Study the drawing (mm; zero at the part's minimum x, y, z) and answer. A direction names the side the tool comes from. Round coordinates to 2 decimals unless told otherwise and drop trailing zeros. Order: outer loops, then holes, each group sorted by start corner. A loop starts at its lowest first (then second) coordinate and runs counter-clockwise, first axis right, second up. Notation, with made-up numbers: (45, -40) -> (64, -40) arc R30 ccw to (64, -5) -> close; hole circle Ø4 at (66, 6). An arc over 180 degrees is marked (long way). Use one line per item in the form item = value.
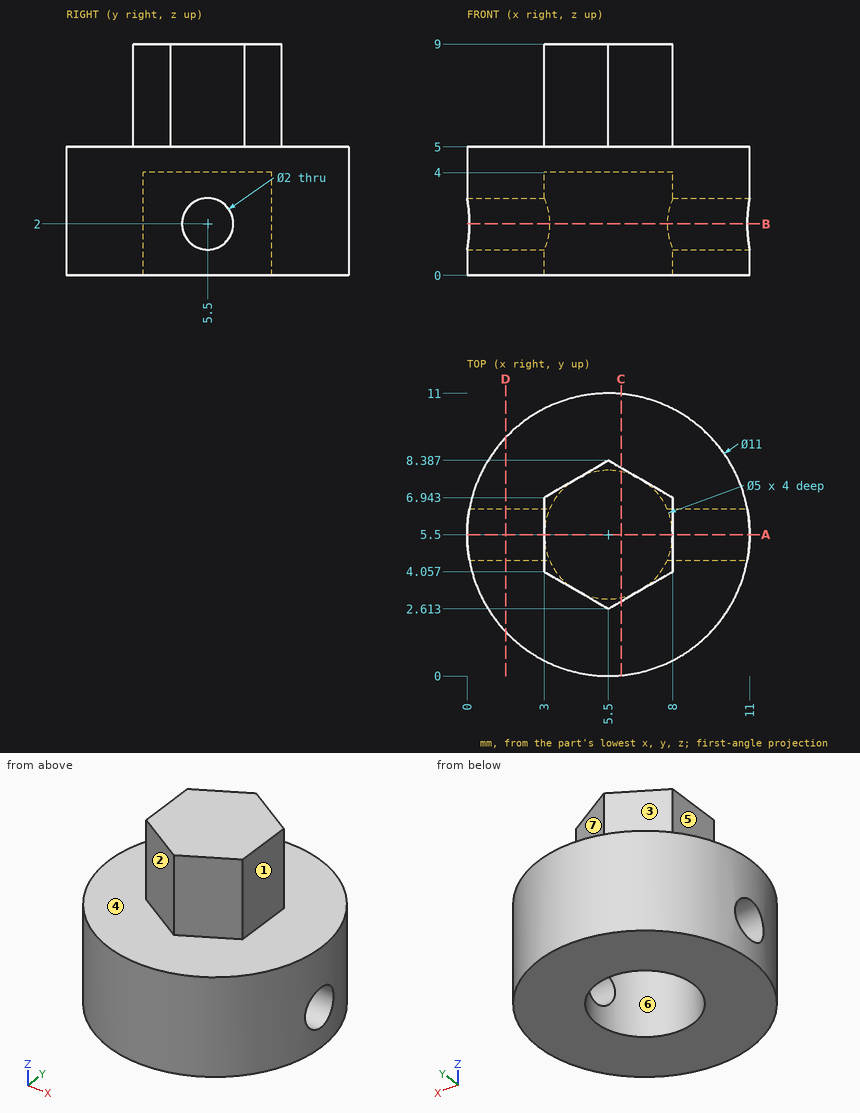
Item 1: Determine the mould class of the marked faces 5, 6 and 7 for opening direction Y: released by +Y, released by -Y, zero draft, split by the parting line, or undercut.
Findings:
face_5 = zero draft
face_6 = undercut
face_7 = released by +Y
Item 2: The part is cut by section A-A, the plane y = 5.5. Give the vertices of the cut face in (x, z), and give its area (3 significant figures).
Findings:
outline = (0, 0) -> (3, 0) -> (3, 1) -> (0, 1) -> close; (0, 3) -> (3, 3) -> (3, 4) -> (8, 4) -> (8, 3) -> (11, 3) -> (11, 5) -> (8, 5) -> (8, 9) -> (3, 9) -> (3, 5) -> (0, 5) -> close; (8, 0) -> (11, 0) -> (11, 1) -> (8, 1) -> close
area = 43.0 mm^2
Item 3: The part is cut by section C-C, the plane x = 6. Give the vertices of the cut face in (y, z).
Findings:
outline = (0.02, 0) -> (3.05, 0) -> (3.05, 4) -> (7.95, 4) -> (7.95, 0) -> (10.98, 0) -> (10.98, 5) -> (8.1, 5) -> (8.1, 9) -> (2.9, 9) -> (2.9, 5) -> (0.02, 5) -> close
Item 4: For the marked faces 1, 2, 3 and 4, determine the directions among +Z, -Z, +X, -X, +Y, -Y from which every point of the face is accessible in a straight line to the end or side of a thin tool.
Findings:
face_1 = +Z, +X, +Y, -Y
face_2 = +Z, -X, -Y
face_3 = +Z, -X, +Y
face_4 = +Z
Item 5: The part is cut by section D-D, the plane x = 1.5. Give the vertices of the cut face in (y, z) (1 decimal), and give its area (3 significant figures).
Findings:
outline = (1.7, 0) -> (9.3, 0) -> (9.3, 5) -> (1.7, 5) -> close; hole circle Ø2 at (5.5, 2)
area = 34.6 mm^2
Item 6: Consider line 1 along Z through (x, y) = (1.1, 5.5); line 2 along Z through (x, y) = (7.25, 9.5); line 3 along X through (y, z) = (6.75, 6.75). Determine where each line is inside the solid, lowest interval first.
Findings:
line_1 = 0 to 1, 3 to 5
line_2 = 0 to 5
line_3 = 3 to 8
Item 7: Flat-ended cylindrical pins translate along their axes: P1, Ø1.5, axis at y = 1.5, z = 4, coming from the -X side; P2, Ø1.4, axis at y = 5.5, z = 6.5, coming from the +X side; P3, Ø1.4, axis at y = 6, z = 7.5, coming from the -X side. Find the tip coordinate at first contact, or state that the pin passes through.
Findings:
P1 = 1.06
P2 = 8
P3 = 3
Item 8: The part is cut by section B-B, the plane z = 2. Give the vertices of the cut face in (x, y).
Findings:
outline = (0.09, 4.5) arc R5.5 ccw to (10.91, 4.5) -> (7.79, 4.5) arc R2.5 cw to (3.21, 4.5) -> close; (0.09, 6.5) -> (3.21, 6.5) arc R2.5 cw to (7.79, 6.5) -> (10.91, 6.5) arc R5.5 ccw to start
